```python
from build123d import *

# Parameters (mm, degrees)
F0_W     = 50
F0_H     = 47.3597366856
F1_DEPTH = 25
F2_R     = 12.5
F3_DEPTH = 25
F5_R     = 0.4552551452


with BuildPart() as f1:
    # F0 (on Top) → F1 (new body)
    with BuildSketch(Plane.XY):
        with Locations((0.0229850411, -3.6821365356)):
            Rectangle(F0_W, F0_H)
    extrude(amount=F1_DEPTH)

    # F2 (on face) → F3 (cut, through all)
    with BuildSketch(Plane.XY.offset(25)):
        Circle(F2_R)
    extrude(amount=-F3_DEPTH, mode=Mode.SUBTRACT)

    # F6: sweep along a path in F4
    with BuildLine(Plane.XY.offset(25)) as f6_path:
        Line((-14.0730467439, -20.5863900483), (16.7477343976, -20.5863900483))
        ThreePointArc((16.7477343976, -20.5863900483), (20.2832683036, -19.1219239542), (21.7477343976, -15.5863900483))
        Line((21.7477343976, -15.5863900483), (21.7477343976, 9.0496650711))
        ThreePointArc((21.7477343976, 9.0496650711), (20.2832683036, 12.585198977), (16.7477343976, 14.0496650711))
        Line((16.7477343976, 14.0496650711), (-14.0730467439, 14.0496650711))
        ThreePointArc((-14.0730467439, 14.0496650711), (-17.6085806498, 12.585198977), (-19.0730467439, 9.0496650711))
        Line((-19.0730467439, 9.0496650711), (-19.0730467439, -15.5863900483))
        ThreePointArc((-19.0730467439, -15.5863900483), (-17.6085806498, -19.1219239542), (-14.0730467439, -20.5863900483))
    # F5 (on Right) → F6 (sweep, cut)
    with BuildSketch(Plane.YZ):
        with Locations((-20.5761548132, 24.9956939369)):
            Circle(F5_R)
    sweep(path=f6_path.line, mode=Mode.SUBTRACT)


solid = f1.part
```
Work out the finished part from the listing and answer in its coordinate system (mm). Give positions to 0.01 mm unless a question says otherwise; leave off trailing zeros. Order: outer loops, then holes, each group sorted by start corner. A loop starts at its lowest first (then second) coordinate and runs counter-clockwise, first axis right, second up. Notation, with made-up numbers: (-25, 45) - (11, 45) arc R20 ccw to (11, 74) - close; hole circle Ø5 at (-4.5, -17.75). An arc over 180 degrees is marked (long way). One line per item, written item: value. Start each with the question number.
1. For a pull along X with two mould halves and no side action, classify faces 1 (the face through (-24.977, -4, 12)), 2 (the face through (0, 19.998, 12)), 3 (the face through (25.023, -4, 12)), 4 (the face through (11.923, 3.755, 12.675)) as released by +X, released by -X, zero draft, split by the parting line, or undercut.
2. Section C-C, the plane z = 16.5 is taken. Write down the section's boundary in (x, y).
3. Section B-B, the plane y = -8.5 is taken. Write down the section's boundary in (x, z).
4. Section A-A, the plane x = 0 is taken. Write down the section's boundary in (y, z), then the cut area to 3 significant figures.
5. Consider line 1 (Y direction, x = 0, z = 18); line 2 (X direction, y = -11.5, z = 19.25); line 3 (X direction, y = 2.5, z = 3). Determine where each line is inside the solid, lowest interval first.
Filled sheet:
1. face 1: released by -X
1. face 2: zero draft
1. face 3: released by +X
1. face 4: undercut
2. outline: (-24.98, -27.36) - (25.02, -27.36) - (25.02, 20) - (-24.98, 20) - close; hole circle Ø25 at (0, 0)
3. outline: (-24.98, 0) - (-9.17, 0) - (-9.17, 25) - (-18.61, 25) arc R0.46 cw (long way) to (-19.52, 25) - (-24.98, 25) - close; (9.17, 0) - (25.02, 0) - (25.02, 25) - (22.19, 25) arc R0.46 cw (long way) to (21.28, 25) - (9.17, 25) - close
4. outline: (-27.36, 0) - (-12.5, 0) - (-12.5, 25) - (-20.12, 25) arc R0.46 cw (long way) to (-21.03, 25) - (-27.36, 25) - close; (12.5, 0) - (20, 0) - (20, 25) - (14.49, 25) arc R0.46 cw (long way) to (13.58, 25) - (12.5, 25) - close
4. area: 558 mm²
5. line 1: -27.36 to -12.5, 12.5 to 20
5. line 2: -24.98 to -4.9, 4.9 to 25.02
5. line 3: -24.98 to -12.25, 12.25 to 25.02
